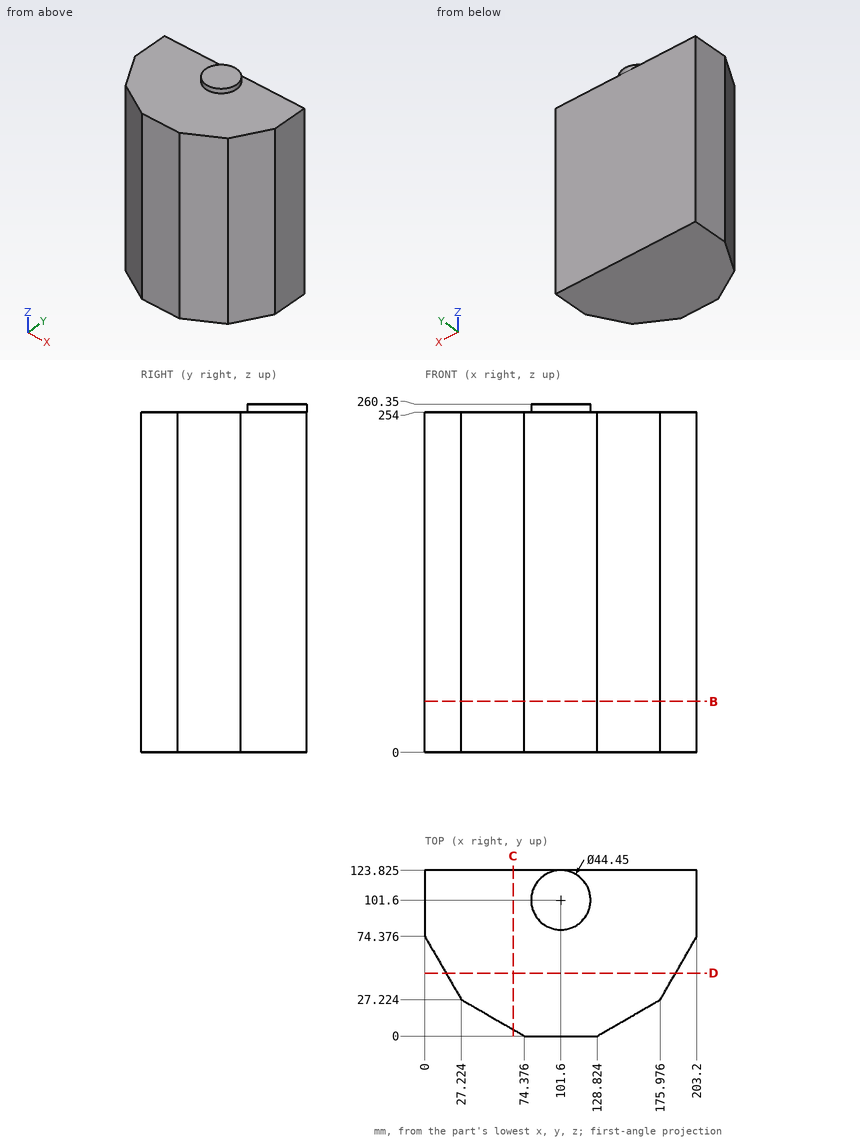
Here's the drawing with two shaded views (mm, measured from the low corner). I have some questions. Coordinates: 2 decimals unless noted, no trailing zeros. Order: outer loops, then holes, each group sorted by start corner. A loop starts at its lowest first (then second) coordinate and runs counter-clockwise, first axis right, second up. Notation, with made-up numbers: (-24.75, 41.5) - (24.25, 41.5) arc R30 cw to (24.25, 70.5) - close; hole circle Ø6 at (-13, -33.75). An arc over 180 degrees is marked (long way). Answer in a Markdown table with one row per item.
1. Suppose I cut it at D-D (y = 47). Please give me the cut outline in (x, z), and give its area (3 significant figures).
Reply:
| item | result |
|---|---|
| outline | (15.81, 0) - (187.39, 0) - (187.39, 254) - (15.81, 254) - close |
| area | 43,600 mm^2 |
2. For pin 1 (4 mm diameter, centred on y = 21, z = 192.5, fed in from -X); pin 2 (1 mm diameter, centred on y = 21.5, z = 114.5, fed in from +X); pin 3 (1 mm diameter, centred on y = 24.5, z = 131, fed in from +X) (1 decimal), each with a flat end and sliding along its axis, tell me the tip position at first contact or that it passes through.
Reply:
| item | result |
|---|---|
| pin 1 | stops at x = 34.54 |
| pin 2 | stops at x = 166.93 |
| pin 3 | stops at x = 172.1 |
3. Suppose I cut it at C-C (x = 66). Please give me the cut outline in (y, z) (1 decimal).
Reply:
| item | result |
|---|---|
| outline | (4.8, 0) - (123.8, 0) - (123.8, 254) - (4.8, 254) - close |
4. Suppose I cut it at B-B (z = 38). Please give me the cut outline in (x, y) (1 decimal), and give its area (3 significant figures).
Reply:
| item | result |
|---|---|
| outline | (0, 74.4) - (27.2, 27.2) - (74.4, 0) - (128.8, 0) - (176, 27.2) - (203.2, 74.4) - (203.2, 123.8) - (0, 123.8) - close |
| area | 21,100 mm^2 |
5. If I drill on line 1 along Z through (x, y) = (83.5, 63); line 2 along Y through (x, z) = (162, 56.5) (1 decimal); line 3 along X through (y, z) = (64, 35), over which ranges is the centre line in solid material (lowest first)?
Reply:
| item | result |
|---|---|
| line 1 | z = 0 to 254 |
| line 2 | y = 19.2 to 123.8 |
| line 3 | x = 5.99 to 197.21 |
